Design review of the part built by this model. Coordinates are the model's own, in mm. A direction names the side the tool comes from. Round coordinates to 2 decimals unless told otherwise and drop trailing zeros. Loops run counter-clockwise (first coordinate to the right, second up) from the corner with the lowest first, then second, coordinate; pieces in that order, holes last. Notation, with made-up numbers: M -27,-3 L -15,-3 A17 cw -15,28 Z; hole C -1.5,1.25 d8. An arc over 180 degrees is marked long. One line per item, written item: value. Start each with the question number.
Item 1: Clearance check with flat-ended pins moving along their axes: pin 1 (3 mm diameter, centred on y = 99.5, z = 90.5, fed in from +X); pin 2 (4 mm diameter, centred on x = -132.57, z = 36.98, fed in from +Y); pin 3 (1.5 mm diameter, centred on x = -131.5, z = 81.5, fed in from -Y). State where each tip first meets the part, or that it passes through.
Item 2: We need section C-C (y = 140). Write out the cut boundary in (x, z).
Item 3: We need section A-A (x = 112.5). Write out the cut boundary in (y, z), then the cut area to 3 significant figures.
Item 4: For line 1 along Y through (x, z) = (93.5, -47); line 2 along X through (y, z) = (46, -89), list the stretches that pass through material, from the lowest coordinate up.
Item 5: We need section D-D (z = -6). Write out the cut boundary in (x, y).
Item 6: For faces 1 (the flat face through (-1, 3, 143)), 2 (the flat face through (-139.124, 79, 2)), list the 3-axis set-ups (+Z, -Z, +X, -X, +Y, -Y) from which the entire face can be reached by the end or side of a thin tool; tool diameter is ignored.
Item 7: We need section B-B (z = -61). Write out the cut boundary in (x, y), then the cut area to 3 significant figures.
from build123d import *

# Parameters (mm, degrees)
SKETCH1_W           = 286
SKETCH1_H           = 286
BOSS_EXTRUDE1_DEPTH = 5
SKETCH4_R           = 2.499853141
SKETCH4_R_2         = 2.499999298
SKETCH4_R_3         = 2.499896797
CUT_EXTRUDE1_DEPTH  = 4
SKETCH5_W           = 286
SKETCH5_H           = 30
CUT_EXTRUDE2_DEPTH  = 203.29434001
SKETCH6_W           = 3.876379433
SKETCH6_H           = 286
BOSS_EXTRUDE2_DEPTH = 150
SKETCH7_W           = 254.74073144
SKETCH7_H           = 20
CUT_EXTRUDE3_DEPTH  = 353.232504579


with BuildPart() as part:
    # Sketch1 → Boss-Extrude1 (new body)
    with BuildSketch(Plane(origin=(0, 0, 0), x_dir=(1, 0, 0), z_dir=(0, 1, 0))):
        Rectangle(SKETCH1_W, SKETCH1_H)
    extrude(amount=BOSS_EXTRUDE1_DEPTH)

    # Sketch4 → Cut-Extrude1 (cut)
    with BuildSketch(Plane(origin=(0, 0, 0), x_dir=(-1, 0, 0), z_dir=(0, -1, 0))):
        with Locations(Location((132.573463178, -80.981198503, 0), (0, 0, 90))):
            Circle(SKETCH4_R)
        with Locations(Location((132.573463178, -36.981198619, 0), (0, 0, 90))):
            Circle(SKETCH4_R_2)
        with Locations(Location((132.569572232, 36.981198719, 0), (0, 0, 90))):
            Circle(SKETCH4_R_3)
        with Locations(Location((132.569572232, 80.981198603, 0), (0, 0, 90))):
            Circle(SKETCH4_R_3)
    extrude(amount=-CUT_EXTRUDE1_DEPTH, mode=Mode.SUBTRACT)

    # Sketch5 → Cut-Extrude2 (cut, through all)
    with BuildSketch(Plane(origin=(0, 5, 0), x_dir=(1, 0, 0), z_dir=(0, 1, 0))):
        Rectangle(SKETCH5_W, SKETCH5_H)
    extrude(amount=-CUT_EXTRUDE2_DEPTH, mode=Mode.SUBTRACT)


with BuildPart() as cut_extrude2_piece_1:
    # of the separate pieces the step leaves, piece 1, a body of its own (cut_extrude2_pieces)
    add(part.part.solids().sort_by_distance((-143, 0, -143))[0])



with BuildPart() as cut_extrude2_piece_2:
    # of the separate pieces the step leaves, piece 2, a body of its own (cut_extrude2_pieces)
    add(part.part.solids().sort_by_distance((-143, 0, 143))[0])


with BuildPart() as cut_extrude2_piece_1_1:
    add(cut_extrude2_piece_1.part)

    add(cut_extrude2_piece_2.part)  # Boss-Extrude2 merges Cut-Extrude2 piece 2
    # Sketch6 → Boss-Extrude2 (add)
    with BuildSketch(Plane(origin=(0, 5, 0), x_dir=(1, 0, 0), z_dir=(0, 1, 0))):
        with Locations((-141.061810283, 0)):
            Rectangle(SKETCH6_W, SKETCH6_H)
    extrude(amount=BOSS_EXTRUDE2_DEPTH)

    # Sketch7 → Cut-Extrude3 (cut, through all)
    with BuildSketch(Plane(origin=(-139.123620567, 0, 0), x_dir=(0, 0, -1), z_dir=(1, 0, 0))):
        with Locations((0, 15)):
            Rectangle(SKETCH7_W, SKETCH7_H)
    extrude(amount=-CUT_EXTRUDE3_DEPTH, mode=Mode.SUBTRACT)


solid = cut_extrude2_piece_1_1.part
A:
1. pin 1: x = -139.12
1. pin 2: y = 5
1. pin 3: y = 4
2. outline: M -143,-143 L -139.12,-143 L -139.12,143 L -143,143 Z
3. outline: M 0,-143 L 5,-143 L 5,-15 L 0,-15 Z; M 0,15 L 5,15 L 5,143 L 0,143 Z
3. area: 1,280 mm2
4. line 1: 0 to 5
4. line 2: -143 to -139.12
5. outline: M -143,25 L -139.12,25 L -139.12,155 L -143,155 Z
6. face 1: +Z, +X, -X, +Y, -Y
6. face 2: +Z, -Z, +X, +Y
7. outline: M -143,0 L 143,0 L 143,5 L -143,5 Z; M -143,25 L -139.12,25 L -139.12,155 L -143,155 Z
7. area: 1,930 mm2
